For this review, take the finished solid that the model builds, in its own axes (mm). Face numbers are marked on the shaded views. A direction names the side the tool comes from. Give positions to 0.01 mm unless a question says otherwise; leave off trailing zeros. Order: outer loops, then holes, each group sorted by start corner. A loop starts at its lowest first (then second) coordinate and runs counter-clockwise, first axis right, second up. Notation, with made-up numbers: (88, 72) -> (98, 72) arc R15 ccw to (98, 83) -> close; hole circle Ø4 at (4, 66). An arc over 180 degrees is marked (long way). Use CSV: the item, a comma, the result in double quotes. Start each with the question number.
```python
from build123d import *

# Parameters (mm, degrees)
BOSS_EXTRUDE1_DEPTH     = 80
CUT_EXTRUDE1_DEPTH      = 96.650405122
CUT_EXTRUDE1_DEPTH_BACK = 96.650405122


with BuildPart() as part:
    # Sketch1 → Boss-Extrude1 (new body)
    with BuildSketch(Plane(origin=(0, 0, 0), x_dir=(1, 0, 0), z_dir=(0, 1, 0))):
        with BuildLine():
            Line((0, -15), (-30, -15))
            Line((-30, -15), (-30, -12.807764064))
            ThreePointArc((-30, -12.807764064), (-27.88205438, -6.65364197), (-22.42535625, -3.106339063))
            Line((-22.42535625, -3.106339063), (-17.57464375, -1.893660937))
            ThreePointArc((-17.57464375, -1.893660937), (-12.11794562, 1.65364197), (-10, 7.807764064))
            Line((-10, 7.807764064), (-10, 43))
            Line((-10, 43), (0, 43))
            Line((0, 43), (10, 43))
            Line((10, 43), (10, 7.807764064))
            ThreePointArc((10, 7.807764064), (12.11794562, 1.65364197), (17.57464375, -1.893660937))
            Line((17.57464375, -1.893660937), (22.42535625, -3.106339063))
            ThreePointArc((22.42535625, -3.106339063), (27.88205438, -6.65364197), (30, -12.807764064))
            Line((30, -12.807764064), (30, -15))
            Line((30, -15), (0, -15))
        make_face()
    extrude(amount=BOSS_EXTRUDE1_DEPTH)

    # Sketch2 → Cut-Extrude1 (cut, two sides: drawn at the far end of the back side and taken through both)
    with BuildSketch(Plane(origin=(0, 0, 0), x_dir=(0, 0, -1), z_dir=(1, 0, 0)).offset(-CUT_EXTRUDE1_DEPTH_BACK)):
        Polygon((237.133104031, 8.5), (43, 8.5), (3, 8.5), (3, 71.5), (43, 71.5), (237.133104031, 71.5), (625.399312092, 71.5), (625.399312092, 8.5), align=None)
    extrude(amount=CUT_EXTRUDE1_DEPTH + CUT_EXTRUDE1_DEPTH_BACK, mode=Mode.SUBTRACT)


solid = part.part
```
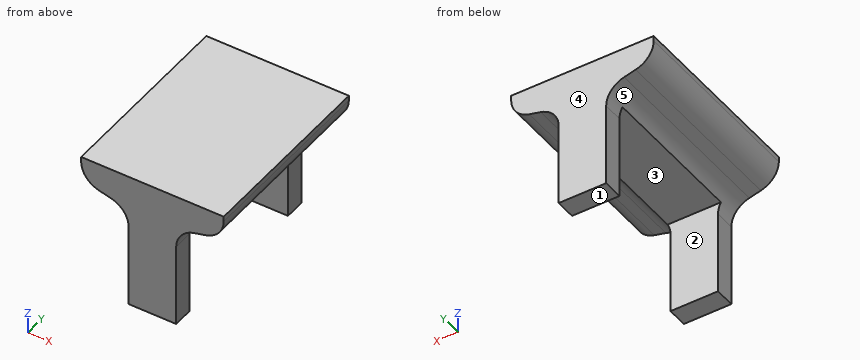
1. For the marked faces 1 and 2, list the 3-axis set-ups (+Z, -Z, +X, -X, +Y, -Y) from which the entire face can be reached by the end or side of a thin tool; tool diameter is ignored.
2. Consider section A-A (z = -35). State the section outline as (x, y) points, plus the area to 3 significant figures.
3. Draft analysis for pull direction Y (two halves, no side actions). For the marked faces 3, 4 and 5, state which applies: +Y half, -Y half, draft (parallel to the pull), parting line (faces both ways), or undercut.
4. To check wall thickness, follow L1, parallel to Y at x = 9.5, z = -28.5; L2, parallel to Z at x = -17.5, y = 66; L3, parallel to Z at x = 0, y = 17. State the ranges of each line that lie inside material, in increasing order. Write a range as [from, to].
5. Consider section B-B (y = 24). State the section outline as (x, z) points.
6. Consider section C-C (x = 5.5). State the section outline as (y, z) points.
7. Clearance check with flat-ended pins moving along their axes: P1, Ø2, axis at y = 36.5, z = 9, coming from the +X side; P2, Ø9.5, axis at y = 75, z = -30.5, coming from the -X side; P3, Ø18, axis at x = -3.5, y = 55.5, coming from the -Z side. State where each tip first meets the part, or that it passes through.
8. Consider section D-D (y = 7). State the section outline as (x, z) points, plus the area to 3 significant figures.
Answer list:
1,face 1,"-Z, +X, -X, +Y, -Y"
1,face 2,"-Z, +X, -X"
2,outline,"(-10, 0) -> (10, 0) -> (10, 8.5) -> (-10, 8.5) -> close; (-10, 71.5) -> (10, 71.5) -> (10, 80) -> (-10, 80) -> close"
2,area,"340 mm2"
3,face 3,"undercut"
3,face 4,"+Y half"
3,face 5,"draft"
4,L1,"[0, 8.5], [71.5, 80]"
4,L2,"[1.87, 15]"
4,L3,"[-3, 15]"
5,outline,"(-30, 12.81) arc R10 ccw to (-22.43, 3.11) -> (-17.57, 1.89) arc R10 cw to (-11.23, -3) -> (11.23, -3) arc R10 cw to (17.57, 1.89) -> (22.43, 3.11) arc R10 ccw to (30, 12.81) -> (30, 15) -> (-30, 15) -> close"
6,outline,"(0, -43) -> (8.5, -43) -> (8.5, -3) -> (71.5, -3) -> (71.5, -43) -> (80, -43) -> (80, 15) -> (0, 15) -> close"
7,P1,"x = 29.6"
7,P2,"x = -10"
7,P3,"z = -3"
8,outline,"(-30, 12.81) arc R10 ccw to (-22.43, 3.11) -> (-17.57, 1.89) arc R10 cw to (-10, -7.81) -> (-10, -43) -> (10, -43) -> (10, -7.81) arc R10 cw to (17.57, 1.89) -> (22.43, 3.11) arc R10 ccw to (30, 12.81) -> (30, 15) -> (-30, 15) -> close"
8,area,"1,660 mm2"
